Input: dimensioned drawing with shaded views. Units: mm. Origin: part minimum x, y, z. A direction names the side the tool comes from. Round coordinates to 2 decimals unless told otherwise and drop trailing zeros. Loops run counter-clockwise (first coordinate to the right, second up) from the corner with the lowest first, then second, coordinate; pieces in that order, holes last. Notation, with made-up numbers: M -40,31.25 L 8,31.25 A25 cw 8,64.25 Z; hole C 77,-8.5 d11. An arc over 180 degrees is marked long. Return JSON: item names as keys, results as strings.
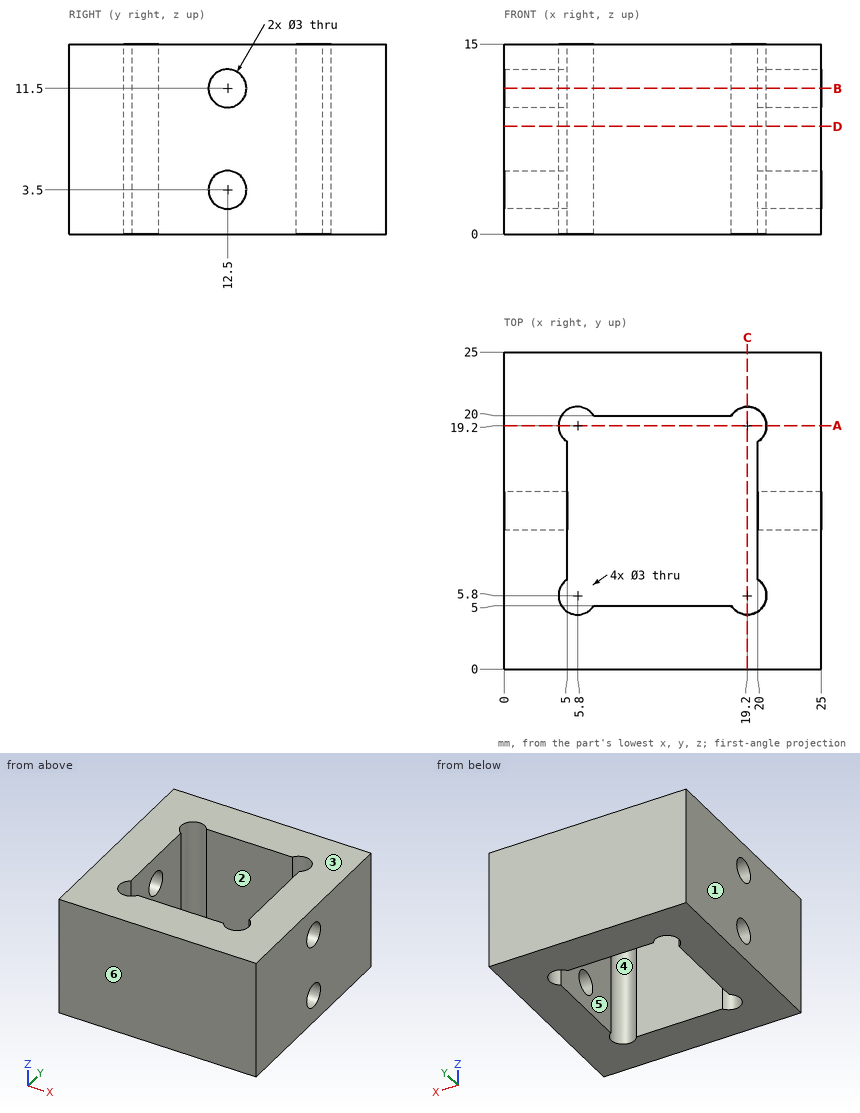
Q1. Section query A-A (y = 19.2). Output: boundary loops of the cut face in (x, z).
Determined:
{"outline": "M 0,0 L 4.3,0 L 4.3,15 L 0,15 Z; M 20.7,0 L 25,0 L 25,15 L 20.7,15 Z"}
Q2. Material intervals for L1, parallel to Y at x = 5.8, z = 6.75; L2, parallel to X at y = 9, z = 10.75, sorted ascending.
Determined:
{"L1": "y = 0 to 4.3, 20.7 to 25", "L2": "x = 0 to 5, 20 to 25"}
Q3. Reachability of the marked faces 5 and 6 from +Z, -Z, +X, -X, +Y, -Y: full face, straight path, thin tool, end or side. Return the list, or none.
Determined:
{"face 5": "+Z, -Z", "face 6": "+Z, -Z, +X, -X, -Y"}
Q4. Section query B-B (z = 11.5). Output: boundary loops of the cut face in (x, y), plus the area to 3 significant figures.
Determined:
{"outline": "M 0,0 L 25,0 L 25,11 L 20,11 L 20,7.07 A1.5 cw long 17.93,5 L 7.07,5 A1.5 cw long 5,7.07 L 5,11 L 0,11 Z; M 0,14 L 5,14 L 5,17.93 A1.5 cw long 7.07,20 L 17.93,20 A1.5 cw long 20,17.93 L 20,14 L 25,14 L 25,25 L 0,25 Z", "area": "360 mm^2"}
Q5. Pull-direction query (X, two-part tool) for the marked faces 1, 2, 3 and 4; classes: pulls with the +X half, pulls with the -X half, needs draft (parallel to the pull), parting line crosses it, or undercut.
Determined:
{"face 1": "pulls with the -X half", "face 2": "undercut", "face 3": "needs draft", "face 4": "undercut"}
Q6. Section query D-D (z = 8.5). Output: boundary loops of the cut face in (x, y).
Determined:
{"outline": "M 0,0 L 25,0 L 25,25 L 0,25 Z; hole M 5,7.07 A1.5 ccw long 7.07,5 L 17.93,5 A1.5 ccw long 20,7.07 L 20,17.93 A1.5 ccw long 17.93,20 L 7.07,20 A1.5 ccw long 5,17.93 Z"}
